Part model, mm, in its own coordinate system. A direction names the side the tool comes from. Round coordinates to 2 decimals unless told otherwise and drop trailing zeros. Loops run counter-clockwise (first coordinate to the right, second up) from the corner with the lowest first, then second, coordinate; pieces in that order, holes last. Notation, with made-up numbers: (-23, -24.5) - (24, -24.5) arc R18 ccw to (24, -9.5) - close; hole circle Ø10 at (18.5, 0.25). An arc over 180 degrees is marked (long way). Put each result on its own line as item: value.
from build123d import *

# Parameters (mm, degrees)
BOSS_EXTRUDE1_DEPTH = 25.4
SKETCH2_R           = 3.2
CUT_EXTRUDE1_DEPTH  = 9


with BuildPart() as part:
    # Sketch1 → Boss-Extrude1 (new body)
    with BuildSketch(Plane.XY):
        with BuildLine():
            Line((124.545, 26.094806075), (132.09, 26.094806075))
            Line((132.09, 26.094806075), (132.09, 8))
            Line((132.09, 8), (159.09, 8))
            Line((159.09, 8), (159.09, 0))
            Line((159.09, 0), (0, 0))
            Line((0, 0), (0, 8))
            Line((0, 8), (27, 8))
            Line((27, 8), (27, 26.094806075))
            Line((27, 26.094806075), (34.545, 26.094806075))
            ThreePointArc((34.545, 26.094806075), (79.545, 5), (124.545, 26.094806075))
        make_face()
    extrude(amount=BOSS_EXTRUDE1_DEPTH)

    # Sketch2 → Cut-Extrude1 (cut, through all)
    with BuildSketch(Plane(origin=(0, 8, 0), x_dir=(1, 0, 0), z_dir=(0, 1, 0))):
        with Locations((8, -12.7)):
            Circle(SKETCH2_R)
        with Locations((151.09, -12.7)):
            Circle(SKETCH2_R)
    extrude(amount=-CUT_EXTRUDE1_DEPTH, mode=Mode.SUBTRACT)


solid = part.part
1. Band-saw the part on A-A (z = 12.7). List the corners of the cut face in (x, y) (3 decimals), plus the area to 3 significant figures.
A:
outline: (0, 0) - (4.8, 0) - (4.8, 8) - (0, 8) - close; (11.2, 0) - (147.89, 0) - (147.89, 8) - (132.09, 8) - (132.09, 26.095) - (124.545, 26.095) arc R58.545 cw to (34.545, 26.095) - (27, 26.095) - (27, 8) - (11.2, 8) - close; (154.29, 0) - (159.09, 0) - (159.09, 8) - (154.29, 8) - close
area: 1,750 mm²
2. Pin check, flat tips, straight feed: P1, Ø9, axis at y = 20, z = 14, coming from the -X side; P2, Ø12.5, axis at x = 147, z = 19, coming from the +Y side; P3, Ø8, axis at x = 46.5, z = 7.5, coming from the +Y side. Stop position of each tip, or through.
A:
P1: stops at x = 27
P2: stops at y = 8
P3: stops at y = 18.21
3. Tool access for faces 4 (the flat face through (128, 26.095, 13)), 5 (the flat face through (145, 8, 13)), 6 (the flat face through (13, 8, 13)): list every direction of +Z, -Z, +X, -X, +Y, -Y with a clear straight run to the whole face (end or side of a thin tool).
A:
face 4: +Z, -Z, +X, -X, +Y
face 5: +Z, -Z, +X, +Y
face 6: +Z, -Z, -X, +Y
4. Band-saw the part on C-C (y = 2.75). List the corners of the cut face in (x, z).
A:
outline: (0, 0) - (159.09, 0) - (159.09, 25.4) - (0, 25.4) - close; hole circle Ø6.4 at (8, 12.7); hole circle Ø6.4 at (151.09, 12.7)
5. Probe line 1 along X through (y, z) = (3.75, 12.7); line 2 along Z through (x, y) = (151.09, 5); line 3 along X through (y, z) = (11.5, 24). List the from-to ranges inside material, lowest first. Write a range as [from, to].
A:
line 1: x = [0, 4.8], [11.2, 147.89], [154.29, 159.09]
line 2: z = [0, 9.5], [15.9, 25.4]
line 3: x = [27, 52.73], [106.36, 132.09]
6. Band-saw the part on D-D (y = 16.25). List the corners of the cut face in (x, z), plus the area to 3 significant figures.
A:
outline: (27, 0) - (45.04, 0) - (45.04, 25.4) - (27, 25.4) - close; (114.05, 0) - (132.09, 0) - (132.09, 25.4) - (114.05, 25.4) - close
area: 916 mm²
7. Band-saw the part on B-B (x = 8). List the corners of the cut face in (y, z), plus the area to 3 significant figures.
A:
outline: (0, 0) - (8, 0) - (8, 9.5) - (0, 9.5) - close; (0, 15.9) - (8, 15.9) - (8, 25.4) - (0, 25.4) - close
area: 152 mm²
8. Two-plate mould, pull along X, no slides. Class faces 1 (the cylindrical face through (78.826, 5.004, 12.522)), 2 (the flat face through (132.09, 17, 13)), 3 (the flat face through (0, 4, 13)): pulls with the +X half, pulls with the -X half, needs draft (parallel to the pull), parting line crosses it, or undercut.
A:
face 1: undercut
face 2: pulls with the +X half
face 3: pulls with the -X half
